from build123d import *

# Parameters (mm, degrees)
CROQUIS1_W              = 42.3
CROQUIS1_H              = 42.3
CROQUIS1_R              = 1.5
SALIENTE_EXTRUIR1_DEPTH = 30
CROQUIS2_R              = 11
SALIENTE_EXTRUIR2_DEPTH = 2
CROQUIS3_R              = 2.5
SALIENTE_EXTRUIR3_DEPTH = 23
CHAFL_N1_SIZE           = 5


with BuildPart() as part:
    # Croquis1 → Saliente-Extruir1 (new, symmetric)
    with BuildSketch(Plane.XY):
        Rectangle(CROQUIS1_W, CROQUIS1_H)
        with Locations((-15.5, 15.5)):
            Circle(CROQUIS1_R, mode=Mode.SUBTRACT)
        with Locations((-15.5, -15.5)):
            Circle(CROQUIS1_R, mode=Mode.SUBTRACT)
        with Locations(Location((15.5, -15.5, 0), (0, 0, 180))):
            Circle(CROQUIS1_R, mode=Mode.SUBTRACT)
        with Locations(Location((15.5, 15.5, 0), (0, 0, 180))):
            Circle(CROQUIS1_R, mode=Mode.SUBTRACT)
    extrude(amount=SALIENTE_EXTRUIR1_DEPTH, both=True)

    # Croquis2 → Saliente-Extruir2 (add)
    with BuildSketch(Plane.XY.offset(30)):
        Circle(CROQUIS2_R)
    extrude(amount=SALIENTE_EXTRUIR2_DEPTH)

    # Croquis3 → Saliente-Extruir3 (add)
    with BuildSketch(Plane.XY.offset(30)):
        Circle(CROQUIS3_R)
    extrude(amount=SALIENTE_EXTRUIR3_DEPTH)

    # Chaflán1
    chafl_n1_edges = [part.edges().sort_by_distance(p)[0] for p in [
        (-21.15, 21.15, 0),
        (21.15, 21.15, 0),
        (21.15, -21.15, 0),
        (-21.15, -21.15, 0),
    ]]
    chamfer(chafl_n1_edges, length=CHAFL_N1_SIZE)


solid = part.part
Work out the finished part from the listing and answer in its coordinate system (mm). A direction names the side the tool comes from. Round coordinates to 2 decimals unless told otherwise and drop trailing zeros. Loops run counter-clockwise (first coordinate to the right, second up) from the corner with the lowest first, then second, coordinate; pieces in that order, holes last. Notation, with made-up numbers: (18.25, -40) - (52.25, -40) arc R33 cw to (52.25, -4) - close; hole circle Ø7 at (7, 26.5). An arc over 180 degrees is marked (long way). One line per item, written item: value.
Q1. Find section B-B on y = 0. Give the vertices of the cut face in (x, z), and give its area (3 significant figures).
Check values:
outline: (-21.15, -30) - (21.15, -30) - (21.15, 30) - (11, 30) - (11, 32) - (2.5, 32) - (2.5, 53) - (-2.5, 53) - (-2.5, 32) - (-11, 32) - (-11, 30) - (-21.15, 30) - close
area: 2,690 mm2
Q2. For faces 1 (the cylindrical face through (-17, -15.43, -0.42)), 2 (the cylindrical face through (-2.38, -10.74, 30.99)), determine the directions among +Z, -Z, +X, -X, +Y, -Y from which every point of the face is accessible in a straight line to the end or side of a thin tool.
Check values:
face 1: +Z, -Z
face 2: +Z
Q3. The mould has two halves that part along X. Classify faces 3 (the cylindrical face through (17, 15.43, -0.42)), 4 (the flat face through (0, 21.15, 0)), 5 (the flat face through (-18.6, -18.7, -0.4)): +X half, -X half, draft (parallel to the pull), parting line (faces both ways), or undercut.
Check values:
face 3: undercut
face 4: draft
face 5: -X half
Q4. Find section A-A on z = 0. Give the vertices of the cut face in (x, y), and give its area (3 significant figures).
Check values:
outline: (-21.15, -16.15) - (-16.15, -21.15) - (16.15, -21.15) - (21.15, -16.15) - (21.15, 16.15) - (16.15, 21.15) - (-16.15, 21.15) - (-21.15, 16.15) - close; hole circle Ø3 at (-15.5, -15.5); hole circle Ø3 at (-15.5, 15.5); hole circle Ø3 at (15.5, -15.5); hole circle Ø3 at (15.5, 15.5)
area: 1,710 mm2
Q5. Find section C-C on x = 6. Give the vertices of the cut face in (y, z).
Check values:
outline: (-21.15, -30) - (21.15, -30) - (21.15, 30) - (9.22, 30) - (9.22, 32) - (-9.22, 32) - (-9.22, 30) - (-21.15, 30) - close
Q6. Find section D-D on z = 44. Give the vertices of the cut face in (x, y), and give its area (3 significant figures).
Check values:
outline: circle Ø5 at (0, 0)
area: 19.6 mm2
Q7. Straight lines are drawn through the part: probe 1 along Y at (x, z) = (-15.5, 0); probe 2 along X at (y, z) = (15, 3). For each, find the intervals that lie inside material, in ascending order.
Check values:
probe 1: -21.15 to -17, -14 to 14, 17 to 21.15
probe 2: -21.15 to -16.91, -14.09 to 14.09, 16.91 to 21.15
Q8. Each of these flat-tipped pins is pushed along its axis until it touches: pin 1 Ø12.5 at (x, y) = (-9, -4) entering from +Z; pin 2 Ø8 at (x, y) = (15, 3) entering from +Z. Where does it stop, or does it pass through?
Check values:
pin 1: z = 32
pin 2: z = 30
